Could you check a few things on this model? Use its own coordinates, in mm. Face numbers are marked on the shaded views. A direction names the side the tool comes from. Give positions to 0.01 mm unless a question says otherwise; leave off trailing zeros. Return JSON: item names as keys, results as strings. Group by question number.
1. If we mould it in two halves opening along X, with no side actions, what happens to the marked faces 1, 2 and 3? For each: +X half, -X half, draft (parallel to the pull), parting line (faces both ways), or undercut.
2. For pin 1 (6 mm diameter, centred on y = 76.5, z = 10.5, fed in from +X); pin 2 (5 mm diameter, centred on x = -48.5, z = 44, fed in from -Y); pin 3 (12 mm diameter, centred on y = -25.5, z = 9, fed in from +X); pin 4 (2 mm diameter, centred on x = -31, y = -59, fed in from -Z), each with a flat end and sliding along its axis, tell me the tip position at first contact or that it passes through.
3. For the marked faces 4 and 5, which set-ups out of +Z, -Z, +X, -X, +Y, -Y let a thin tool reach every point of the face, with its end or its side?
4. If we section it at A-A (y = -62.5): State how many separate pieces and enclosed holes the cut face has, plus the area to 3 significant figures.
5. Please list where these lines run through material, in increasing order: line 1 (Y direction, x = -60, z = 8); line 2 (Y direction, x = 35, z = 6.5); line 3 (Y direction, x = -69, z = 47.5).
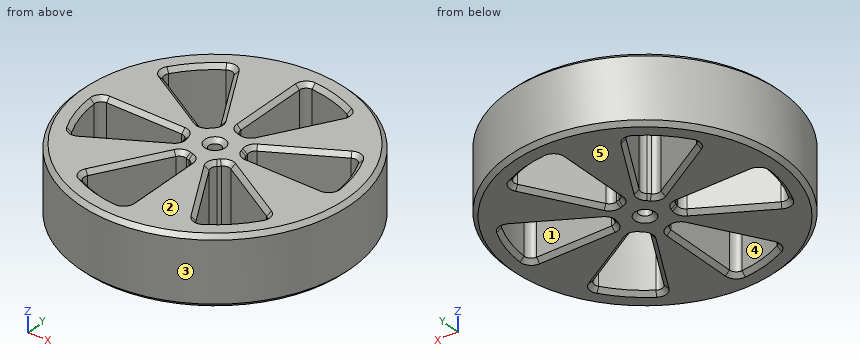
```python
from build123d import *

# Parameters (mm, degrees)
SKETCH1_R           = 100
BOSS_EXTRUDE1_DEPTH = 50
CUT_EXTRUDE1_DEPTH  = 151
CIRPATTERN1_COUNT   = 6
FILLET1_R           = 5
SKETCH3_R           = 4.5
CUT_EXTRUDE2_DEPTH  = 151
CHAMFER1_SIZE       = 3


with BuildPart() as part:
    # Sketch1 → Boss-Extrude1 (new body)
    with BuildSketch(Plane.XY):
        Circle(SKETCH1_R)
    extrude(amount=BOSS_EXTRUDE1_DEPTH)

    # Sketch2 → Cut-Extrude1 (cut, through all)
    with BuildSketch(Plane.XY.offset(50)):
        with BuildLine():
            Line((0, 85), (0, 20))
            ThreePointArc((0, 20), (5.176380902, 19.318516526), (10, 17.320508076))
            Line((10, 17.320508076), (42.5, 73.612159322))
            ThreePointArc((42.5, 73.612159322), (21.999618834, 82.103695235), (0, 85))
        make_face()
    cut_extrude1 = extrude(amount=-CUT_EXTRUDE1_DEPTH, mode=Mode.SUBTRACT)

    # CirPattern1: Cut-Extrude1 ×6 about axis
    cirpattern1_axis = Axis((0, 0, 0), (0, 0, 1))
    for i in range(1, CIRPATTERN1_COUNT):
        add(cut_extrude1.rotate(cirpattern1_axis, i * 360 / CIRPATTERN1_COUNT), mode=Mode.SUBTRACT)

    # Fillet1
    fillet1_edges = [part.edges().sort_by_distance(p)[0] for p in [
        (42.5, 73.612159322, 25),
        (10, 17.320508076, 25),
        (0, 20, 25),
        (0, 85, 25),
        (85, 0, 25),
        (20, 0, 25),
        (17.320508076, 10, 25),
        (73.612159322, 42.5, 25),
        (42.5, -73.612159322, 25),
        (10, -17.320508076, 25),
        (17.320508076, -10, 25),
        (73.612159322, -42.5, 25),
        (-85, 0, 25),
        (-20, 0, 25),
        (-17.320508076, -10, 25),
        (-73.612159322, -42.5, 25),
        (-42.5, -73.612159322, 25),
        (-10, -17.320508076, 25),
        (0, -20, 25),
        (0, -85, 25),
        (-42.5, 73.612159322, 25),
        (-10, 17.320508076, 25),
        (-17.320508076, 10, 25),
        (-73.612159322, 42.5, 25),
    ]]
    fillet(fillet1_edges, radius=FILLET1_R)

    # Sketch3 → Cut-Extrude2 (cut, through all)
    with BuildSketch(Plane.XY.offset(50)):
        Circle(SKETCH3_R)
    extrude(amount=-CUT_EXTRUDE2_DEPTH, mode=Mode.SUBTRACT)

    # Chamfer1
    chamfer1_edges = [part.edges().sort_by_distance(p)[0] for p in [
        (21.999618834, 82.103695235, 50),
        (21.999618834, 82.103695235, 0),
        (26.084623635, 45.179893433, 50),
        (26.084623635, 45.179893433, 0),
        (5.176380902, 19.318516526, 50),
        (5.176380902, 19.318516526, 0),
        (-14.142135624, 14.142135624, 50),
        (-14.142135624, 14.142135624, 0),
        (-45.179893433, 26.084623635, 50),
        (-45.179893433, 26.084623635, 0),
        (-60.104076401, 60.104076401, 50),
        (-60.104076401, 60.104076401, 0),
        (-26.084623635, 45.179893433, 50),
        (-26.084623635, 45.179893433, 0),
        (-5.176380902, -19.318516526, 50),
        (-5.176380902, -19.318516526, 0),
        (0, -52.169247271, 50),
        (0, -52.169247271, 0),
        (-21.999618834, -82.103695235, 50),
        (-21.999618834, -82.103695235, 0),
        (-26.084623635, -45.179893433, 50),
        (-26.084623635, -45.179893433, 0),
        (-19.318516526, -5.176380902, 50),
        (-19.318516526, -5.176380902, 0),
        (-45.179893433, -26.084623635, 50),
        (-45.179893433, -26.084623635, 0),
        (-82.103695235, -21.999618834, 50),
        (-82.103695235, -21.999618834, 0),
        (-52.169247271, 0, 50),
        (-52.169247271, 0, 0),
        (14.142135624, -14.142135624, 50),
        (14.142135624, -14.142135624, 0),
        (45.179893433, -26.084623635, 50),
        (45.179893433, -26.084623635, 0),
        (60.104076401, -60.104076401, 50),
        (60.104076401, -60.104076401, 0),
        (26.084623635, -45.179893433, 50),
        (26.084623635, -45.179893433, 0),
        (19.318516526, 5.176380902, 50),
        (19.318516526, 5.176380902, 0),
        (45.179893433, 26.084623635, 50),
        (45.179893433, 26.084623635, 0),
        (82.103695235, 21.999618834, 50),
        (82.103695235, 21.999618834, 0),
        (52.169247271, 0, 50),
        (52.169247271, 0, 0),
        (1.576734016, 83.487942048, 50),
        (1.576734016, 83.487942048, 0),
        (40.378479311, 73.091045731, 50),
        (40.378479311, 73.091045731, 0),
        (9.690284831, 19.038098975, 50),
        (9.690284831, 19.038098975, 0),
        (-17.911082321, 11.642334937, 50),
        (-17.911082321, 11.642334937, 0),
        (-71.514311715, 43.109462736, 50),
        (-71.514311715, 43.109462736, 0),
        (-43.109462736, 71.514311715, 50),
        (-43.109462736, 71.514311715, 0),
        (-11.642334937, 17.911082321, 50),
        (-11.642334937, 17.911082321, 0),
        (-1.127016654, -21.332619768, 50),
        (-1.127016654, -21.332619768, 0),
        (-1.576734016, -83.487942048, 50),
        (-1.576734016, -83.487942048, 0),
        (-40.378479311, -73.091045731, 50),
        (-40.378479311, -73.091045731, 0),
        (-9.690284831, -19.038098975, 50),
        (-9.690284831, -19.038098975, 0),
        (-19.038098975, -9.690284831, 50),
        (-19.038098975, -9.690284831, 0),
        (-73.091045731, -40.378479311, 50),
        (-73.091045731, -40.378479311, 0),
        (-83.487942048, -1.576734016, 50),
        (-83.487942048, -1.576734016, 0),
        (-21.332619768, -1.127016654, 50),
        (-21.332619768, -1.127016654, 0),
        (17.911082321, -11.642334937, 50),
        (17.911082321, -11.642334937, 0),
        (71.514311715, -43.109462736, 50),
        (71.514311715, -43.109462736, 0),
        (43.109462736, -71.514311715, 50),
        (43.109462736, -71.514311715, 0),
        (11.642334937, -17.911082321, 50),
        (11.642334937, -17.911082321, 0),
        (19.038098975, 9.690284831, 50),
        (19.038098975, 9.690284831, 0),
        (73.091045731, 40.378479311, 50),
        (73.091045731, 40.378479311, 0),
        (83.487942048, 1.576734016, 50),
        (83.487942048, 1.576734016, 0),
        (21.332619768, 1.127016654, 50),
        (21.332619768, 1.127016654, 0),
        (1.127016654, 21.332619768, 50),
        (1.127016654, 21.332619768, 0),
        (-100, 0, 0),
        (-4.5, 0, 0),
        (-4.5, 0, 50),
        (-100, 0, 50),
        (0, 52.169247271, 50),
        (0, 52.169247271, 0),
    ]]
    chamfer(chamfer1_edges, length=CHAMFER1_SIZE)


solid = part.part
```
Answer:
{
 "1": {"face 1": "undercut", "face 2": "draft", "face 3": "parting line"},
 "2": {"pin 1": "stops at x = 67.81", "pin 2": "stops at y = -88.79", "pin 3": "stops at x = 98.08", "pin 4": "passes through"},
 "3": {"face 4": "+Z, -Z", "face 5": "-Z, +X, -X, +Y, -Y"},
 "4": {"separate pieces": "3", "enclosed holes": "0", "area": "4,860 mm²"},
 "5": {"line 1": "y = -80 to -34.64, 0 to 34.64, 60.21 to 80", "line 2": "y = -93.67 to -60.62, -20.21 to 0, 20.21 to 60.62, 77.46 to 93.67", "line 3": "y = -71.69 to -40.41, 0.5 to 39.26, 50.49 to 71.69"}
}
